Autodesk Inventor part; units mm, degrees
ref_plane "YZ Plane" through (0, 0, 0) normal (1, 0, 0) x (0, 1, 0)
ref_plane "XZ Plane" through (0, 0, 0) normal (0, 1, 0) x (-1, 0, 0)
ref_plane "XY Plane" through (0, 0, 0) normal (0, 0, 1) x (1, 0, 0)
sketch "Sketch1" plane through (0, 0, 0) normal (0, 1, 0) x (-1, 0, 0)
  line L0 (0, 0) -> (60, 0)
  line L1 (60, 0) -> (60, -45)
  line L2 (60, -45) -> (0, -45)
  line L3 (0, -45) -> (0, 0)
  dimension "d0" = 60
  dimension "d1" = 45
extrude "Extrusion1" add sketch "Sketch1" along normal blind 5
sketch "Sketch2" plane through (0, 5, 0) normal (0, 1, 0) x (1, 0, 0)
  line L0 (-60, 0) -> (0, 0)
  line L1 (0, 0) -> (0, 45)
  line L2 (0, 45) -> (-60, 45)
  line L3 (-60, 45) -> (-60, 0)
  circle A0 centre (-8, 36.3) radius 4
  line L4 (-24.9532, 22.5) -> (-60, 22.5)
  circle A1 centre (-8, 8.7) radius 4
  dimension "d5" = 45
  dimension "d7" = 8
  dimension "d8" = 8.7
  dimension "d10" = 8
extrude "Extrusion3" cut sketch "Sketch2" against normal up to next contours A0 | A1
equation "\"d7\" = d4"
equation "\"d10\" = d9"
equation "\"d6\" = d4"
equation "\"d9\" = d6"
properties part number "MotorFixer"
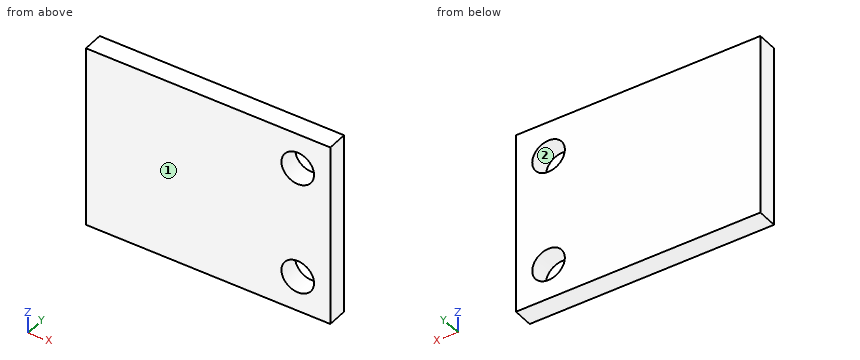
Source: CAD feature listing. Evaluate the final solid. Frame: model axes, mm. Face numbers are marked on the shaded views. Coordinates: 2 decimals unless noted, no trailing zeros. Loops run counter-clockwise (first coordinate to the right, second up) from the corner with the lowest first, then second, coordinate; pieces in that order, holes last. Notation, with made-up numbers: M 39.25,-39.75 L 74.25,-39.75 A15 cw 74.25,-32.75 Z; hole C -34,56.5 d4. An arc over 180 degrees is marked long. Use a Markdown table: item, result. Add a question column.
Q1. Material intervals for L1, parallel to Z at x = -8, y = 1.85; L2, parallel to X at y = 3.4, z = -8.7; L3, parallel to X at y = 3.6, z = -40, sorted ascending.
Q2. Section query A-A, the plane z = -36.3. Return loops of the section in (x, y).
Q3. Section query B-B, the plane x = -8. Return loops of the section in (y, z), and give its area (3 significant figures).
Q4. Draft query along X for the marked faces 1 and 2. Return one class per face: pulls with the +X half, pulls with the -X half, needs draft (parallel to the pull), parting line crosses it, or undercut.
Q5. First-contact query: pin 1 (6.5 mm diameter, centred on x = -8, z = -36.3, fed in from +Y). Flat tip, straight axial feed; report the tip coordinate or a pass-through.
Q6. Section query C-C, the plane y = 3.1. Return loops of the section in (x, z).
Result:
| question | item | result |
|---|---|---|
| 1 | L1 | z = -45 to -40.3, -32.3 to -12.7, -4.7 to 0 |
| 1 | L2 | x = -60 to -12, -4 to 0 |
| 1 | L3 | x = -60 to -9.52, -6.48 to 0 |
| 2 | outline | M -60,0 L -12,0 L -12,5 L -60,5 Z; M -4,0 L 0,0 L 0,5 L -4,5 Z |
| 3 | outline | M 0,-45 L 5,-45 L 5,-40.3 L 0,-40.3 Z; M 0,-32.3 L 5,-32.3 L 5,-12.7 L 0,-12.7 Z; M 0,-4.7 L 5,-4.7 L 5,0 L 0,0 Z |
| 3 | area | 145 mm2 |
| 4 | face 1 | needs draft |
| 4 | face 2 | undercut |
| 5 | pin 1 | passes through |
| 6 | outline | M -60,-45 L 0,-45 L 0,0 L -60,0 Z; hole C -8,-36.3 d8; hole C -8,-8.7 d8 |
